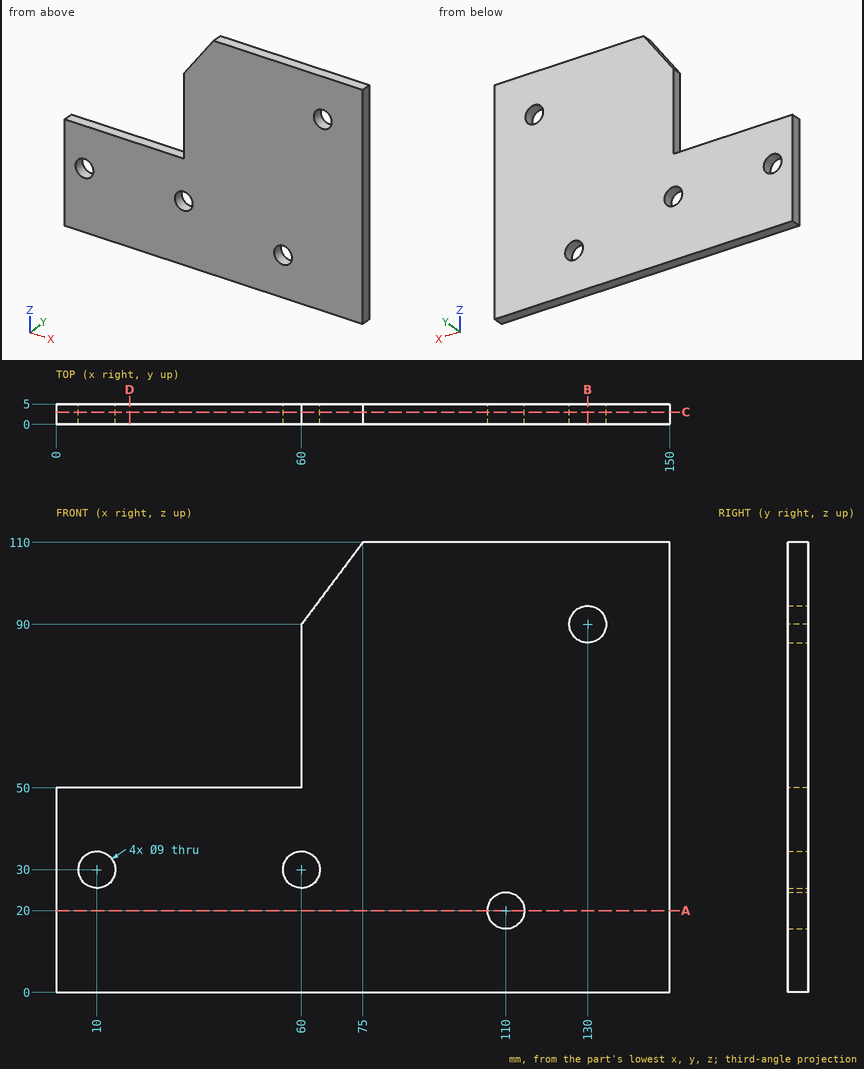
Verification items for this drawing (mm, ordinates from the low corner). Coordinates: 2 decimals unless noted, no trailing zeros. Order: outer loops, then holes, each group sorted by start corner. A loop starts at its lowest first (then second) coordinate and runs counter-clockwise, first axis right, second up. Notation, with made-up numbers: M 14,51.25 L 32,51.25 A18 ccw 32,70.25 Z; hole C -21.5,-28.5 d2. An arc over 180 degrees is marked long. Write each question's results on one line, items separated by ' | '.
1) Section check A-A on z = 20. Record the cut outline in (x, y).
Solved:
outline: M 0,0 L 105.5,0 L 105.5,5 L 0,5 Z; M 114.5,0 L 150,0 L 150,5 L 114.5,5 Z
2) Section check B-B on x = 130. Record the cut outline in (y, z).
Solved:
outline: M 0,0 L 5,0 L 5,85.5 L 0,85.5 Z; M 0,94.5 L 5,94.5 L 5,110 L 0,110 Z
3) Gauge pin test, flat ends, axial feed: pin 1 Ø7 at (x, z) = (110, 20) entering from +Y; pin 2 Ø2.5 at (x, y) = (25, 3.5) entering from +Z. Record the tip position at first contact, or that the pin passes through.
Solved:
pin 1: passes through | pin 2: stops at z = 50
4) Section check D-D on x = 18. Record the cut outline in (y, z).
Solved:
outline: M 0,0 L 5,0 L 5,50 L 0,50 Z
5) Section check C-C on y = 3. Record the cut outline in (x, z), plus the area to 3 significant figures.
Solved:
outline: M 0,0 L 150,0 L 150,110 L 75,110 L 60,90 L 60,50 L 0,50 Z; hole C 10,30 d9; hole C 60,30 d9; hole C 110,20 d9; hole C 130,90 d9 | area: 12,500 mm²
6) Scan lines: line 1 along X through (y, z) = (4.35, 26); line 2 along Z through (x, y) = (10, 3.2); line 3 along Z through (x, y) = (127.5, 3.7). Record each from-to range of solid material in increasing order. Write a range as [from, to].
Solved:
line 1: x = [0, 7.94], [12.06, 57.94], [62.06, 150] | line 2: z = [0, 25.5], [34.5, 50] | line 3: z = [0, 86.26], [93.74, 110]
